Geometry: see drawing. Coordinates: mm, zero at the bounding-box minimum. A direction names the side the tool comes from. Coordinates: 2 decimals unless noted, no trailing zeros. Write each loop counter-clockwise with the first axis right and the second up, starting at its lowest first coordinate (ties: lowest second). Pieces come first, ordered by that corner, then holes.
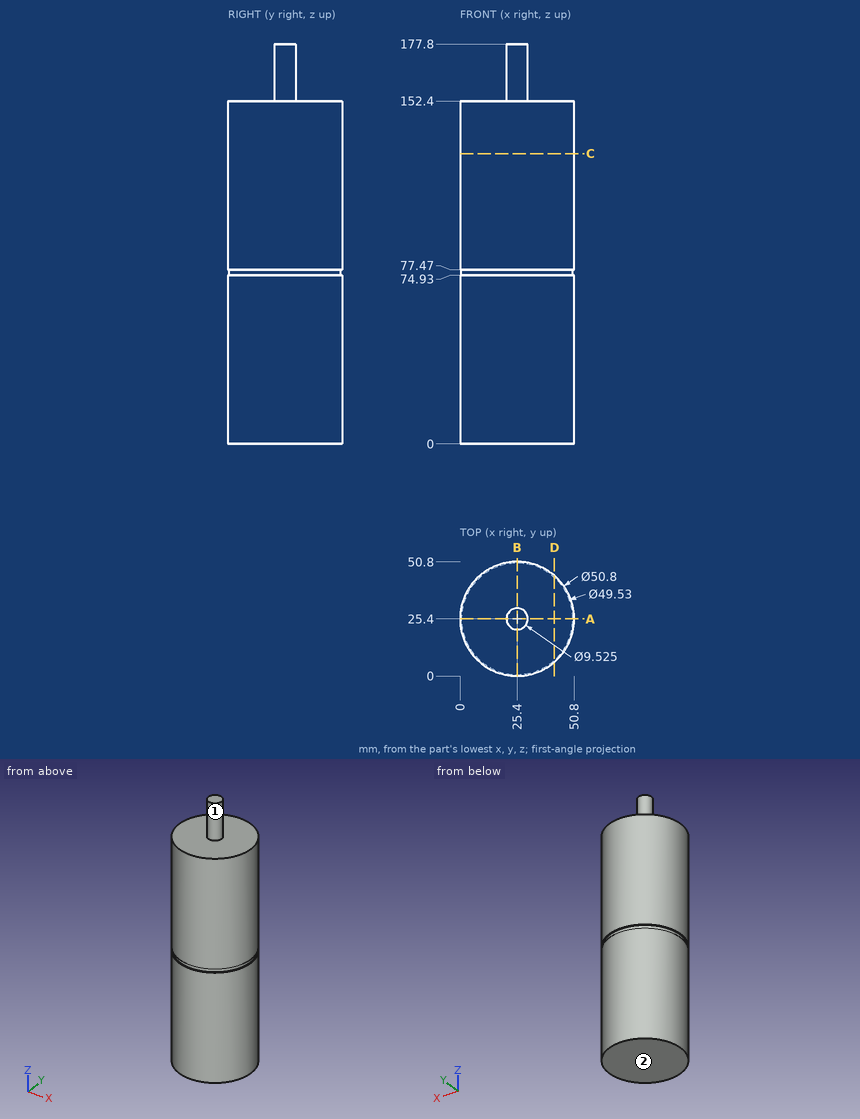
Item 1: Section C-C, the plane z = 129. Output: boundary loops of the cut face in (x, y), plus the area to 3 significant figures.
Derived:
outline: circle Ø50.8 at (25.4, 25.4)
area: 2,030 mm2
Item 2: Section A-A, the plane y = 25.4. Output: boundary loops of the cut face in (x, z) (1 decimal), plus the area to 3 significant figures.
Derived:
outline: (0, 0) - (50.8, 0) - (50.8, 74.9) - (50.2, 74.9) - (50.2, 77.5) - (50.8, 77.5) - (50.8, 152.4) - (30.2, 152.4) - (30.2, 177.8) - (20.6, 177.8) - (20.6, 152.4) - (0, 152.4) - (0, 77.5) - (0.6, 77.5) - (0.6, 74.9) - (0, 74.9) - close
area: 7,980 mm2
Item 3: Pin query (flat end, axial travel): pin 1 (4 mm diameter, centred on x = 44, z = 39, fed in from -Y) (3 decimals); pin 2 (3 mm diameter, centred on x = 11.5, z = 133, fed in from -Y); pin 3 (2 mm diameter, centred on y = 33, z = 83, fed in from +X). Return the tip coordinate at first contact, or that it passes through.
Derived:
pin 1: stops at y = 6.175
pin 2: stops at y = 3.23
pin 3: stops at x = 49.93
Item 4: Section D-D, the plane x = 42. Output: boundary loops of the cut face in (y, z), plus the area to 3 significant figures.
Derived:
outline: (6.18, 0) - (44.62, 0) - (44.62, 74.93) - (43.78, 74.93) - (43.78, 77.47) - (44.62, 77.47) - (44.62, 152.4) - (6.18, 152.4) - (6.18, 77.47) - (7.02, 77.47) - (7.02, 74.93) - (6.18, 74.93) - close
area: 5,860 mm2
Item 5: Set-up query: the marked faces 1 and 2. Return all of +Z, -Z, +X, -X, +Y, -Y with unobstructed straight access to the full face (end or side cutting, diameter ignored); none if empty.
Derived:
face 1: +Z
face 2: -Z, +X, -X, +Y, -Y
Item 6: Material intervals for probe 1 along Z at (x, y) = (34, 48.5); probe 2 along X at (y, z) = (25.5, 47); probe 3 along Y at (x, z) = (26.5, 31), sorted ascending.
Derived:
probe 1: z = 0 to 152.4
probe 2: x = 0 to 50.8
probe 3: y = 0.02 to 50.78
